Part model, mm, in its own coordinate system. Coordinates: 2 decimals unless noted, no trailing zeros. Loops run counter-clockwise (first coordinate to the right, second up) from the corner with the lowest first, then second, coordinate; pieces in that order, holes last. Notation, with made-up numbers: M 78,85.25 L 126,85.25 A17 cw 126,111.25 Z; hole C -13.5,13.25 d10. An arc over 180 degrees is marked long. Use a Markdown table: item, result. Add a question column.
1) Band-saw the part on C-C (z = 10). List the corners of the cut face in (x, y).
2) Wall check: probe 1 along Z at (x, y) = (180, -2.55); probe 2 along Z at (x, y) = (0, -2); probe 3 along X at (y, z) = (-0.8, 2.5). Give the ranges that are in metal, low to high. Write a range as from..to.
3) Band-saw the part on A-A (y = -2.75). List the corners of the cut face in (x, z).
4) Pull direction X, two halves, no side cores. Call faces 1 (the flat face through (55, -4, 0)), 2 (the cylindrical face through (183.815, -1.972, 1.54)), 3 (the cylindrical face through (187.5, -2, 0.2)): released by +X, released by -X, zero draft, split by the parting line, or undercut.
5) Band-saw the part on B-B (x = 76.5). List the corners of the cut face in (y, z), plus the area to 3 significant figures.
6) Pin check, flat tips, straight feed: pin 1 Ø2 at (y, z) = (-3, -4.5) entering from -X; pin 2 Ø10.5 at (x, z) = (0, 0) entering from +Y; pin 3 Ø7 at (x, z) = (180, 0.339) entering from +Y; pin 4 Ø1 at (y, z) = (-0.5, 3) entering from +X. Stop position of each tip, or through.
from build123d import *

# Parameters (mm, degrees)
F0_R     = 4
F1_DEPTH = 4


with BuildPart() as f1:
    # F0 (on Front) → F1 (new body)
    with BuildSketch(Plane.XZ):
        with BuildLine():
            Line((-0.894263, 12.467971), (-67.350288, 7.701424))
            ThreePointArc((-67.350288, 7.701424), (-74.313689, 0.245409), (-67.399684, -7.256434))
            Line((-67.399684, -7.256434), (-0.97659, -12.461793))
            ThreePointArc((-0.97659, -12.461793), (-0.303359, -12.496318), (0.370754, -12.4945))
            Line((0.370754, -12.4945), (180.222452, -7.1577))
            ThreePointArc((180.222452, -7.1577), (187.499987, 0.353125), (180.194213, 7.836485))
            Line((180.194213, 7.836485), (0.323688, 12.495808))
            ThreePointArc((0.323688, 12.495808), (-0.285627, 12.496736), (-0.894263, 12.467971))
        make_face()
        with Locations((-66.81373, 0.220642)):
            Circle(F0_R, mode=Mode.SUBTRACT)
        Circle(F0_R, mode=Mode.SUBTRACT)
        with Locations((180, 0.339)):
            Circle(F0_R, mode=Mode.SUBTRACT)
    extrude(amount=F1_DEPTH)


solid = f1.part
Entries:
| question | item | result |
|---|---|---|
| 1 | outline | M -35.3,-4 L 96.67,-4 L 96.67,0 L -35.3,0 Z |
| 2 | probe 1 | -7.16..-3.66, 4.34..7.84 |
| 2 | probe 2 | -12.5..-4, 4..12.5 |
| 2 | probe 3 | -73.96..-70.1, -63.53..-3.12, 3.12..176.63, 183.37..187.18 |
| 3 | outline | M -67.4,-7.26 L -0.98,-12.46 A12.5 ccw 0.37,-12.49 L 180.22,-7.16 A7.5 ccw 180.19,7.84 L 0.32,12.5 A12.5 ccw -0.89,12.47 L -67.35,7.7 A7.5 ccw Z; hole C -66.81,0.22 d8; hole C 0,0 d8; hole C 180,0.34 d8 |
| 4 | face 1 | zero draft |
| 4 | face 2 | undercut |
| 4 | face 3 | released by +X |
| 5 | outline | M -4,-10.24 L 0,-10.24 L 0,10.52 L -4,10.52 Z |
| 5 | area | 83.0 mm2 |
| 6 | pin 1 | x = -73.33 |
| 6 | pin 2 | y = 0 |
| 6 | pin 3 | through |
| 6 | pin 4 | x = 187.18 |
